The listing builds one solid part. Answer for the finished solid, in the listing's coordinates (mm). Face numbers are marked on the shaded views. A direction names the side the tool comes from. Coordinates: 2 decimals unless noted, no trailing zeros. Loops run counter-clockwise (first coordinate to the right, second up) from the corner with the lowest first, then second, coordinate; pieces in that order, holes last. Notation, with made-up numbers: M 86,5 L 126,5 A24 ccw 126,44 Z; hole C 54,0.5 d10. An arc over 180 degrees is marked long. Answer in a Markdown table with one row per item. Add a question column.
from build123d import *

# Parameters (mm, degrees)
BOSS_EXTRU_1_DEPTH = 25.5
BOSS_EXTRU_2_DEPTH = 5
BOSS_EXTRU_3_DEPTH = 5
BOSS_EXTRU_4_DEPTH = 5
BOSS_EXTRU_5_DEPTH = 5
ESQUISSE6_W        = 4.8
ESQUISSE6_H        = 31
ESQUISSE7_W        = 2.9
ESQUISSE7_H        = 35
PER_AGE1_D         = 3.18
PER_AGE1_DEPTH     = 5
PER_AGE2_D         = 3.18
PER_AGE3_D         = 3.18
PER_AGE3_DEPTH     = 5
PER_AGE4_D         = 3.18
CONG_1_R           = 1
CONG_2_R           = 2
CONG_3_R           = 3


with BuildPart() as part:
    # Esquisse1 → Boss.-Extru.1 (new body)
    with BuildSketch(Plane(origin=(12.75, 0, 0), x_dir=(0, 0, -1), z_dir=(1, 0, 0))):
        Polygon((-5, -2.5), (0, -12.5), (0, 12.5), (-5, 2.5), align=None)
    extrude(amount=-BOSS_EXTRU_1_DEPTH)

    # Esquisse2 → Boss.-Extru.2 (add)
    with BuildSketch(Plane(origin=(-12.75, 0, 0), x_dir=(0, -1, 0), z_dir=(-1, 0, 0))):
        Polygon((4.5, 16), (4.5, 4), (12.5, 0), (12.5, 16), align=None)
    extrude(amount=-BOSS_EXTRU_2_DEPTH)

    # Esquisse3 → Boss.-Extru.3 (add)
    with BuildSketch(Plane(origin=(12.75, 0, 0), x_dir=(0, 0, -1), z_dir=(1, 0, 0))):
        Polygon((-16, -12.5), (0, -12.5), (-4, -4.5), (-16, -4.5), align=None)
    extrude(amount=-BOSS_EXTRU_3_DEPTH)

    # Esquisse4 → Boss.-Extru.4 (add)
    with BuildSketch(Plane(origin=(12.75, 0, 0), x_dir=(0, 0, -1), z_dir=(1, 0, 0))):
        Polygon((-16, 4.5), (-4, 4.5), (0, 12.5), (-16, 12.5), align=None)
    extrude(amount=-BOSS_EXTRU_4_DEPTH)

    # Esquisse5 → Boss.-Extru.5 (add)
    with BuildSketch(Plane(origin=(-12.75, 0, 0), x_dir=(0, -1, 0), z_dir=(-1, 0, 0))):
        Polygon((-4.5, 16), (-12.5, 16), (-12.5, 0), (-4.5, 4), align=None)
    extrude(amount=-BOSS_EXTRU_5_DEPTH)

    # Esquisse6 → Révolution1 (revolve)
    with BuildSketch(Plane(origin=(0, 0, 0), x_dir=(1, 0, 0), z_dir=(0, 1, 0))):
        with Locations((2.4, 15.5)):
            Rectangle(ESQUISSE6_W, ESQUISSE6_H)
    revolve(axis=Axis((0, 0, -31), (0, 0, 1)))

    # Esquisse7 → Révolution2 (revolve)
    with BuildSketch(Plane(origin=(0.009791841, 0, -27.999996576), x_dir=(0.999999938851933, 0, 0.0003497086364192443), z_dir=(-0.0003497086364192443, 0, 0.999999938851933)), mode=Mode.PRIVATE) as r_volution2_sk:
        with Locations((-1.459791842, 21.3249183)):
            Rectangle(ESQUISSE7_W, ESQUISSE7_H)
    revolve(r_volution2_sk.sketch.rotate(Axis((0, 3.8249183, -28), (0, 1, 0)), 90.020036829), axis=Axis((0, 3.8249183, -28), (0, 1, 0)))

    # Perçage1
    with Locations(Plane.ZY.offset(12.75)):
        with Locations((12, -8.5)):
            Hole(PER_AGE1_D / 2, depth=PER_AGE1_DEPTH)

    # Perçage2 (through all)
    with Locations(Plane.ZY.offset(-7.75)):
        with Locations((12, -8.5)):
            Hole(PER_AGE2_D / 2)

    # Perçage3
    with Locations(Plane(origin=(12.75, 0, 0), x_dir=(0, 0, -1), z_dir=(1, 0, 0))):
        with Locations((-12, 8.5)):
            Hole(PER_AGE3_D / 2, depth=PER_AGE3_DEPTH)

    # Perçage4 (through all)
    with Locations(Plane(origin=(-7.75, 0, 0), x_dir=(0, 0, -1), z_dir=(1, 0, 0))):
        with Locations((-12, 8.5)):
            Hole(PER_AGE4_D / 2)

    # Congé1
    cong_1_edges = [part.edges().sort_by_distance(p)[0] for p in [
        (12.75, 0, 5),
        (-12.75, 0, 5),
        (0, -2.5, 5),
        (0, 2.5, 5),
    ]]
    fillet(cong_1_edges, radius=CONG_1_R - 0.0001)  # a hair under: the kernel refuses the full size

    # Congé2
    cong_2_edges = [part.edges().sort_by_distance(p)[0] for p in [
        (-7.75, -8.5, 2),
        (7.75, -8.5, 2),
        (7.75, 8.5, 2),
        (-7.75, 8.5, 2),
        (-4.8, 0, 0),
    ]]
    fillet(cong_2_edges, radius=CONG_2_R)

    # Congé3
    cong_3_edges = [part.edges().sort_by_distance(p)[0] for p in [
        (-10.25, -4.5, 16),
        (-10.25, -12.5, 16),
        (10.25, -12.5, 16),
        (10.25, -4.5, 16),
        (10.25, 4.5, 16),
        (10.25, 12.5, 16),
        (-10.25, 4.5, 16),
        (-10.25, 12.5, 16),
    ]]
    fillet(cong_3_edges, radius=CONG_3_R)


solid = part.part
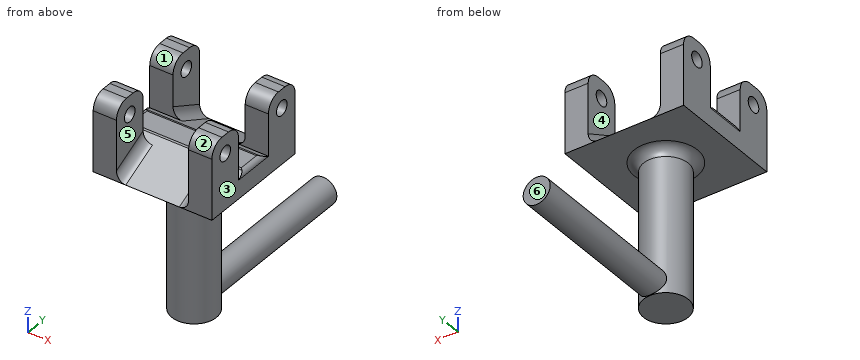
(1) A cutting plane is placed at A-A (z = 12). State how many separate pieces and enclosed holes the cut face has, plus the area to 3 significant figures.
(2) The mould has two halves that part along X. Classify the marked faces 3, 4, 5 and 6: released by +X, released by -X, zero draft, split by the parting line, or undercut.
(3) For the marked faces 1 and 2, determine the directions among +Z, -Z, +X, -X, +Y, -Y from which every point of the face is accessible in a straight line to the end or side of a thin tool.
(4) Each of these flat-tipped pins is pushed along its axis until it touches: pin 1 (4 mm diameter, centred on x = -8.5, z = 1, fed in from +Y); pin 2 (1.5 mm diameter, centred on x = -8.5, y = -1.5, fed in from -Z); pin 3 (4 mm diameter, centred on x = 2.5, y = 17, fed in from +Z). Where does it stop, or does it pass through?
(5) Straight lines are drawn through the part: line 1 (Y direction, x = 11.6, z = 12); line 2 (Y direction, x = 10.5, z = 0.5); line 3 (Y direction, x = 0, z = -15.5). For each, find the intervals that lie inside material, in ascending order.
(6) A cutting plane is placed at C-C (x = 0). Give the vertices of the cut face in (y, z), plus the area to 3 significant figures.
(7) A cutting plane is placed at B-B (y = 0). Give the vertices of the cut face in (x, z).
Solved:
| question | item | result |
|---|---|---|
| 1 | separate pieces | 8 |
| 1 | enclosed holes | 0 |
| 1 | area | 96.4 mm² |
| 2 | face 3 | released by +X |
| 2 | face 4 | undercut |
| 2 | face 5 | undercut |
| 2 | face 6 | zero draft |
| 3 | face 1 | +Z, +X, -X |
| 3 | face 2 | +Z, +X, -X, -Y |
| 4 | pin 1 | stops at y = 12.5 |
| 4 | pin 2 | stops at z = 0 |
| 4 | pin 3 | stops at z = -25.14 |
| 5 | line 1 | y = -12.5 to -10.09, -6.91 to -4.5, 4.5 to 6.91, 10.09 to 12.5 |
| 5 | line 2 | y = -12.5 to 12.5 |
| 5 | line 3 | y = -4.8 to 4.8 |
| 6 | outline | M -12.5,0 L -6.8,0 A2 cw -4.8,-2 L -4.8,-31 L 4.8,-31 L 4.8,-30.9 L 38.82,-30.9 L 38.82,-25.1 L 4.8,-25.1 L 4.8,-2 A2 cw 6.8,0 L 12.5,0 L 2.71,4.89 A1 ccw 2.26,5 L -2.26,5 A1 ccw -2.71,4.89 Z |
| 6 | area | 572 mm² |
| 7 | outline | M -12.75,0 L -6.8,0 A2 cw -4.8,-2 L -4.8,-31 L 4.8,-31 L 4.8,-2 A2 cw 6.8,0 L 12.75,0 L 12.75,4 A1 ccw 11.75,5 L -11.75,5 A1 ccw -12.75,4 Z |
